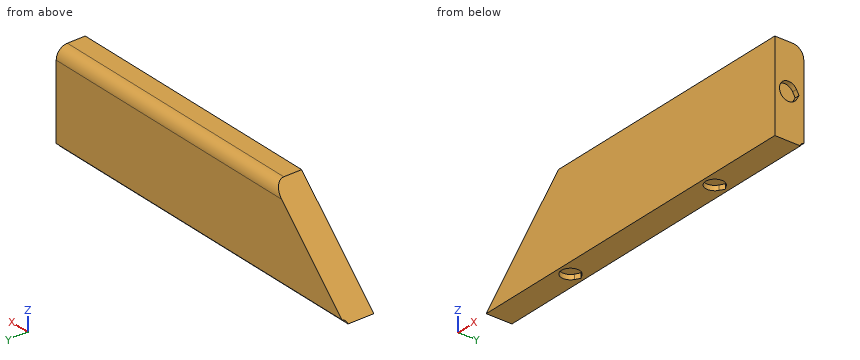
from build123d import *

# Parameters (mm, degrees)
EXTRUDE_1_DEPTH     = 13
SWEEP_START         = -80
SWEEP_1_DEPTH       = 160
SKETCH_6_R          = 4.075
CUT_EXTRUDE_1_DEPTH = 2.15
FILLET_1_R          = 5
SKETCH_7_R          = 4.075
CUT_EXTRUDE_2_DEPTH = 2.15


# Read off the part's stored shape, not the designer's step: Вырез-По траектории1
with BuildPart() as part:
    # Эскиз1 → Бобышка-Вытянуть1 (new body)
    with BuildSketch(Plane(origin=(0, 0, 0), x_dir=(1, 0, 0), z_dir=(0, 1, 0))):
        Polygon((-40, -20), (80, -20), (80, 20), (-80, 20), align=None)
    extrude(amount=-EXTRUDE_1_DEPTH)

    # Вырез-По траектории1 outline → Вырез-По траектории1 (cut)
    with BuildSketch(Plane.YZ.offset(SWEEP_START)):
        with BuildLine():
            ThreePointArc((0, -18.5), (-1.060660172, -18.939339828), (-1.5, -20))
            Line((-1.5, -20), (0, -20))
            Line((0, -20), (0, -18.5))
        make_face()
    extrude(amount=SWEEP_1_DEPTH, mode=Mode.SUBTRACT)

    # Эскиз6 → Вырез-Вытянуть1 (cut)
    with BuildSketch(Plane(origin=(0, 0, -20), x_dir=(-1, 0, 0), z_dir=(0, 0, -1))):
        with Locations((-40, -7.565202347)):
            Circle(SKETCH_6_R)
        with BuildLine():
            Line((-40, -2.859797653), (-42.0375, -4.036148827))
            ThreePointArc((-42.0375, -4.036148827), (-40, -3.490202347), (-37.9625, -4.036148827))
            Line((-37.9625, -4.036148827), (-40, -2.859797653))
        make_face()
        with Locations((40, -7.565202347)):
            Circle(SKETCH_6_R)
        with BuildLine():
            ThreePointArc((37.9625, -4.036148827), (40, -3.490202347), (42.0375, -4.036148827))
            Line((42.0375, -4.036148827), (40, -2.859797653))
            Line((40, -2.859797653), (37.9625, -4.036148827))
        make_face()
    extrude(amount=-CUT_EXTRUDE_1_DEPTH, mode=Mode.SUBTRACT)

    # Скругление1
    fillet_1_edges = [part.edges().sort_by_distance(p)[0] for p in [
        (20, 0, 20),
    ]]
    fillet(fillet_1_edges, radius=FILLET_1_R)

    # Эскиз7 → Вырез-Вытянуть2 (cut)
    with BuildSketch(Plane.ZY.offset(-80)):
        with Locations((0, -6.815202347)):
            Circle(SKETCH_7_R)
        with BuildLine():
            Line((2.0375, -3.286148827), (0, -2.109797653))
            Line((0, -2.109797653), (-2.0375, -3.286148827))
            ThreePointArc((-2.0375, -3.286148827), (0, -2.740202347), (2.0375, -3.286148827))
        make_face()
    extrude(amount=CUT_EXTRUDE_2_DEPTH, mode=Mode.SUBTRACT)


solid = part.part
Input: part model. Units: mm. Frame: model coordinates. Give positions to 0.01 mm unless a question says otherwise; leave off trailing zeros. Loops run counter-clockwise (first coordinate to the right, second up) from the corner with the lowest first, then second, coordinate; pieces in that order, holes last. Notation, with made-up numbers: M 70,17.5 L 121,17.5 A12 ccw 121,23.5 Z; hole C 25.25,72.25 d11. An arc over 180 degrees is marked long. Use CSV: the item, a comma, the result in double quotes.
(1) Section B-B, the plane y = -8.75. Return loops of the section in (x, z).
Outcome:
outline,"M -80,-20 L -43.9,-20 L -43.9,-17.85 L -36.1,-17.85 L -36.1,-20 L 36.1,-20 L 36.1,-17.85 L 43.9,-17.85 L 43.9,-20 L 80,-20 L 80,-3.59 L 77.85,-3.59 L 77.85,3.59 L 80,3.59 L 80,20 L -40,20 Z"
(2) Pin query (flat end, axial travel): P1, Ø2.5, axis at y = -5, z = 2, coming from the +X side; P2, Ø2.5, axis at x = 40.5, y = -8.5, coming from the -Z side; P3, Ø4, axis at y = -5, z = 7, coming from the -X side. Return the tip coordinate at first contact, or that it passes through.
Outcome:
P1,"stops at x = 77.85"
P2,"stops at z = -17.85"
P3,"stops at x = -55"
(3) Section C-C, the plane z = 8.5. Return loops of the section in (x, y), plus the area to 3 significant figures.
Outcome:
outline,"M -51.5,-13 L 80,-13 L 80,0 L -51.5,0 Z"
area,"1,710 mm²"
(4) Material intervals for L1, parallel to Y at x = -40, z = -18.45; L2, parallel to Y at x = 78.5, z = 0; L3, parallel to Z at x = -37, y = -7.75, sorted ascending. Write a range as [from, to].
Outcome:
L1,"y = [-13, -11.64], [-2.86, 0]"
L2,"y = [-13, -10.89], [-2.11, 0]"
L3,"z = [-17.85, 20]"
(5) Section A-A, the plane x = -47. Return loops of the section in (y, z), plus the area to 3 significant figures.
Outcome:
outline,"M -13,-20 L -1.5,-20 A1.5 cw 0,-18.5 L 0,13 L -13,13 Z"
area,"427 mm²"
